```python
from build123d import *

# Parameters (mm, degrees)
F0_W     = 175
F0_H     = 85
F1_DEPTH = 65
F2_R     = 40
F3_DEPTH = 5
F4_R     = 2.38125
F5_DEPTH = 10


with BuildPart() as f1:
    # F0 (on Top) → F1 (new body)
    with BuildSketch(Plane.XY):
        Rectangle(F0_W, F0_H)
    extrude(amount=F1_DEPTH)

    # F2 (on face) → F3 (cut)
    with BuildSketch(Plane.XY.offset(65)):
        with Locations((30.3, 0)):
            Circle(F2_R)
    extrude(amount=-F3_DEPTH, mode=Mode.SUBTRACT)

    # F4 (on face) → F5 (cut)
    with BuildSketch(Plane(origin=(-87.5, 0, 0), x_dir=(0, -1, 0), z_dir=(-1, 0, 0))):
        with Locations((-33.5, 12.8)):
            Circle(F4_R)
        with Locations((-33.5, 56.8)):
            Circle(F4_R)
        with Locations((37.3, 28.8)):
            Circle(F4_R)
    extrude(amount=-F5_DEPTH, mode=Mode.SUBTRACT)


solid = f1.part
```
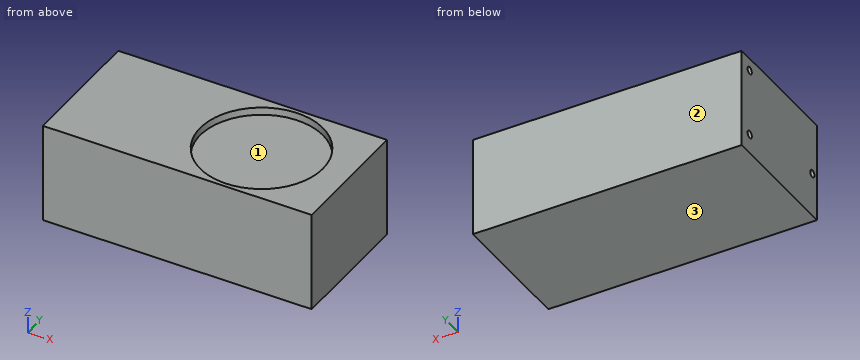
Input: part model. Units: mm. Frame: model coordinates. Face numbers are marked on the shaded views. Give positions to 0.01 mm unless a question says otherwise; leave off trailing zeros. Write each loop counter-clockwise with the first axis right and the second up, starting at its lowest first coordinate (ties: lowest second). Pieces come first, ordered by that corner, then holes. Notation, with made-up numbers: (60, 42.25) - (68, 42.25) arc R19 cw to (68, 50.25) - close; hole circle Ø7 at (79, 70). An arc over 180 degrees is marked (long way). Write item = value, one per line. Start each with the question number.
1) Draft query along Y for the marked faces 1, 2 and 3. Return one class per face: pulls with the +Y half, pulls with the -Y half, needs draft (parallel to the pull), parting line crosses it, or undercut.
2) Pin query (flat end, axial travel): pin 1 (4 mm diameter, centred on x = 51, y = 18.5, fed in from +Z); pin 2 (1.4 mm diameter, centred on y = -36.5, z = 30, fed in from -X). Return the tip coordinate at first contact, or that it passes through.
3) Cut plane A-A (y = 0). Return loops of the section in (x, z), and give its area (3 significant figures).
4) Material intervals for L1, parallel to Z at x = -85.5, y = 33.5; L2, parallel to Y at x = 30, z = 61; L3, parallel to Z at x = -81, y = 33, sorted ascending. Write a range as [from, to].
5) Cut plane D-D (y = 33.5). Return loops of the section in (x, z).
6) Cut plane C-C (y = -37.3). Return loops of the section in (x, z).
7) Cut plane B-B (y = -19.5). Return loops of the section in (x, z), and give its area (3 significant figures).
Answers follow:
q1.face_1 = undercut
q1.face_2 = pulls with the +Y half
q1.face_3 = needs draft
q2.pin_1 = 60
q2.pin_2 = -77.5
q3.outline = (-87.5, 0) - (87.5, 0) - (87.5, 65) - (70.3, 65) - (70.3, 60) - (-9.7, 60) - (-9.7, 65) - (-87.5, 65) - close
q3.area = 11,000 mm^2
q4.L1 = [0, 10.42], [15.18, 54.42], [59.18, 65]
q4.L2 = [-42.5, -40], [40, 42.5]
q4.L3 = [0, 10.47], [15.13, 54.47], [59.13, 65]
q5.outline = (-87.5, 0) - (87.5, 0) - (87.5, 65) - (52.16, 65) - (52.16, 60) - (8.44, 60) - (8.44, 65) - (-87.5, 65) - (-87.5, 59.18) - (-77.5, 59.18) - (-77.5, 54.42) - (-87.5, 54.42) - (-87.5, 15.18) - (-77.5, 15.18) - (-77.5, 10.42) - (-87.5, 10.42) - close
q6.outline = (-87.5, 0) - (87.5, 0) - (87.5, 65) - (44.75, 65) - (44.75, 60) - (15.85, 60) - (15.85, 65) - (-87.5, 65) - (-87.5, 31.18) - (-77.5, 31.18) - (-77.5, 26.42) - (-87.5, 26.42) - close
q7.outline = (-87.5, 0) - (87.5, 0) - (87.5, 65) - (65.22, 65) - (65.22, 60) - (-4.62, 60) - (-4.62, 65) - (-87.5, 65) - close
q7.area = 11,000 mm^2
